Verification items for the finished model (mm, model axes). A direction names the side the tool comes from. Round coordinates to 2 decimals unless told otherwise and drop trailing zeros. Order: outer loops, then holes, each group sorted by start corner. A loop starts at its lowest first (then second) coordinate and runs counter-clockwise, first axis right, second up. Notation, with made-up numbers: (-6.75, 46) -> (43.25, 46) arc R32 cw to (43.25, 83) -> close; hole circle Ø9 at (45, 44.25). An arc over 180 degrees is marked (long way). Answer in a Markdown table with one row per item. Add a question column.
```python
from build123d import *

# Parameters (mm, degrees)
SKETCH025_W             = 22.5
SKETCH025_H             = 16.5
PAD012_DEPTH            = 3.5
SKETCH026_R             = 2.2
POCKET009_DEPTH         = 2
SKETCH027_R             = 1
POCKET010_DEPTH         = 3.501
SKETCH028_W             = 17.3
SKETCH028_H             = 7.9
PAD013_DEPTH            = 17
BODY003_PLACEMENT_ANGLE = 180


with BuildPart() as part:
    # Sketch025 → Pad012 (new body)
    with BuildSketch(Plane.XZ):
        with Locations((11.25, 8.25)):
            Rectangle(SKETCH025_W, SKETCH025_H)
    extrude(amount=PAD012_DEPTH)

    # Sketch026 (on Face6 of Pad012) → Pocket009 (cut)
    with BuildSketch(Plane.XZ.offset(3.5)):
        with Locations((4.45, 13.25)):
            Circle(SKETCH026_R)
        with Locations((18.05, 13.25)):
            Circle(SKETCH026_R)
    extrude(amount=-POCKET009_DEPTH, mode=Mode.SUBTRACT)

    # Sketch027 (on Face5 of Pocket009) → Pocket010 (cut, through all)
    with BuildSketch(Plane.XZ.offset(3.5)):
        with Locations((4.45, 13.25)):
            Circle(SKETCH027_R)
        with Locations((18.05, 13.25)):
            Circle(SKETCH027_R)
    extrude(amount=-POCKET010_DEPTH, mode=Mode.SUBTRACT)

    # Sketch028 (on Face4 of Pocket010) → Pad013 (join)
    with BuildSketch(Plane(origin=(0, 0, 0), x_dir=(1, 0, 0), z_dir=(0, 1, 0))):
        with Locations((11.25, -6.8)):
            Rectangle(SKETCH028_W, SKETCH028_H)
    extrude(amount=PAD013_DEPTH)


with BuildPart() as part_1:
    # Body003 placement: moved
    add(part.part.moved(Location((29.2, 70.5, -0.5))).rotate(Axis((29.2, 70.5, -0.5), (0, 0, 1)), BODY003_PLACEMENT_ANGLE))


solid = part_1.part
```
1) Cross-section at A-A, the plane z = 12.75. Record the boundary of the cut face in (x, y).
2) Depth check by flat-ended pin: P1, Ø6, axis at x = 11, y = 61.5, coming from the -Z side; P2, Ø12, axis at x = 23, y = 57.5, coming from the +Z side; P3, Ø4, axis at y = 59.5, z = 5.5, coming from the +X side. Enter the tip coordinate at first touch or a pass-through.
3) Draft check along X on faces 6 (the face through (24.967, 71.261, 11.774)), 7 (the face through (9.3, 62, 6)), 8 (the face through (29.2, 72, 8)), 9 (the face through (18, 62, 2.35)). Enter one of: +X half, -X half, draft (parallel to the pull), parting line (faces both ways), or undercut.
4) Cross-section at B-B, the plane x = 24.75. Record the boundary of the cut face in (y, z), and give its area (3 significant figures).
5) Cross-section at C-C, the plane z = 2.75. Record the boundary of the cut face in (x, y), and give its area (3 significant figures).
6) Cross-section at D-D, the plane x = 21.25. Record the boundary of the cut face in (y, z).
7) Thickness scan on L1, parallel to Z at x = 24.75, y = 72.5; L2, parallel to X at y = 68.25, z = 3.5; L3, parallel to Y at x = 21.75, z = 13.5. Record the ranges inside material, lowest first. Write a range as [from, to].
8) Tool access check on faces 1 (the face through (12.77, 73.01, 14.24)), 2 (the face through (26.6, 62, 6)), 3 (the face through (18, 53.5, 6)), 4 (the face through (10.226, 71.261, 12.367)), 5 (the face through (18, 62, 10.25)). Record the directions out of +Z, -Z, +X, -X, +Y, -Y that give a thin tool (end or side, any length) a straight path to the whole face; none if there is none.
Results below:
| question | item | result |
|---|---|---|
| 1 | outline | (6.7, 70.5) -> (10.15, 70.5) -> (10.15, 72) -> (8.95, 72) -> (8.95, 74) -> (6.7, 74) -> close; (12.15, 70.5) -> (23.75, 70.5) -> (23.75, 72) -> (22.55, 72) -> (22.55, 74) -> (13.35, 74) -> (13.35, 72) -> (12.15, 72) -> close; (25.75, 70.5) -> (29.2, 70.5) -> (29.2, 74) -> (26.95, 74) -> (26.95, 72) -> (25.75, 72) -> close |
| 2 | P1 | z = 2.35 |
| 2 | P2 | z = 10.25 |
| 2 | P3 | x = 26.6 |
| 3 | face 6 | undercut |
| 3 | face 7 | -X half |
| 3 | face 8 | +X half |
| 3 | face 9 | draft |
| 4 | outline | (53.5, 2.35) -> (70.5, 2.35) -> (70.5, -0.5) -> (74, -0.5) -> (74, 10.55) -> (72, 10.55) -> (72, 11.75) -> (70.5, 11.75) -> (70.5, 10.25) -> (53.5, 10.25) -> close; (70.5, 13.75) -> (72, 13.75) -> (72, 14.95) -> (74, 14.95) -> (74, 16) -> (70.5, 16) -> close |
| 4 | area | 180 mm² |
| 5 | outline | (6.7, 70.5) -> (9.3, 70.5) -> (9.3, 53.5) -> (26.6, 53.5) -> (26.6, 70.5) -> (29.2, 70.5) -> (29.2, 74) -> (6.7, 74) -> close |
| 5 | area | 373 mm² |
| 6 | outline | (53.5, 2.35) -> (70.5, 2.35) -> (70.5, -0.5) -> (74, -0.5) -> (74, 16) -> (70.5, 16) -> (70.5, 10.25) -> (53.5, 10.25) -> close |
| 7 | L1 | [-0.5, 10.55], [14.95, 16] |
| 7 | L2 | [9.3, 26.6] |
| 7 | L3 | [70.5, 74] |
| 8 | face 1 | +Y |
| 8 | face 2 | +Z, -Z, +X, -Y |
| 8 | face 3 | +Z, -Z, +X, -X, -Y |
| 8 | face 4 | +Y, -Y |
| 8 | face 5 | +Z, +X, -X, -Y |
